from build123d import *

# Parameters (mm, degrees)
SKETCH_1_R      = 1.05
EXTRUDE_1_DEPTH = 1.5
FILLET_1_R      = 1


with BuildPart() as part:
    # 草图1 → 凸台-拉伸1 (new body)
    with BuildSketch(Plane.XY):
        Polygon((23.32, 41.958612035), (27.19, 41.958612035), (27.19, 46.958612035), (24.99, 46.958612035), (24.99, 48.458612035), (29.39, 48.458612035), (29.39, 46.958612035), (28.69, 46.958612035), (28.69, 41.958612035), (33.69, 41.958612035), (33.69, 56.958612035), (14.32, 56.958612035), (-5.05, 56.958612035), (-5.05, 41.958612035), (-0.05, 41.958612035), (-0.05, 46.958612035), (-0.75, 46.958612035), (-0.75, 48.458612035), (3.65, 48.458612035), (3.65, 46.958612035), (1.45, 46.958612035), (1.45, 41.958612035), (5.32, 41.958612035), (5.32, 50.958612035), (23.32, 50.958612035), align=None)
        with Locations((27.94, 53.458612035)):
            Circle(SKETCH_1_R, mode=Mode.SUBTRACT)
        with Locations(Location((0.7, 53.458612035, 0), (0, 0, 180))):
            Circle(SKETCH_1_R, mode=Mode.SUBTRACT)
    extrude(amount=EXTRUDE_1_DEPTH)

    # 圆角1
    fillet_1_edges = [part.edges().sort_by_distance(p)[0] for p in [
        (-5.05, 41.958612035, 0.75),
        (-5.05, 56.958612035, 0.75),
        (33.69, 56.958612035, 0.75),
        (33.69, 41.958612035, 0.75),
        (23.32, 41.958612035, 0.75),
        (5.32, 41.958612035, 0.75),
    ]]
    fillet(fillet_1_edges, radius=FILLET_1_R)


solid = part.part
Input: part model. Units: mm. Frame: model coordinates. A direction names the side the tool comes from. Coordinates: 2 decimals unless noted, no trailing zeros. Loops run counter-clockwise (first coordinate to the right, second up) from the corner with the lowest first, then second, coordinate; pieces in that order, holes last. Notation, with made-up numbers: (12.25, 27.5) -> (64.25, 27.5) arc R23 ccw to (64.25, 43.5) -> close; hole circle Ø9 at (26.25, 14.5). An arc over 180 degrees is marked (long way). One line per item, written item: value.
(1) Set-up query: faces 5 (the face through (24.99, 48, 1)), 6 (the face through (5.32, 47, 1)), 7 (the face through (-4.75, 56.67, 0.76)). Return all of +Z, -Z, +X, -X, +Y, -Y with unobstructed straight access to the full face (end or side cutting, diameter ignored); none if empty.
Answer below:
face 5: +Z, -Z
face 6: +Z, -Z, -Y
face 7: +Z, -Z, -X, +Y
(2) Draft query along X for faces 1 (the face through (-0.05, 44, 1)), 2 (the face through (33.69, 49, 1)), 3 (the face through (-5.05, 50, 1)), 4 (the face through (31, 41.959, 1)). Return one class per face: pulls with the +X half, pulls with the -X half, needs draft (parallel to the pull), parting line crosses it, or undercut.
Answer below:
face 1: undercut
face 2: pulls with the +X half
face 3: pulls with the -X half
face 4: needs draft
(3) Cut plane A-A (y = 46.25). Output: boundary loops of the cut face in (x, z).
Answer below:
outline: (-5.05, 0) -> (-0.05, 0) -> (-0.05, 1.5) -> (-5.05, 1.5) -> close; (1.45, 0) -> (5.32, 0) -> (5.32, 1.5) -> (1.45, 1.5) -> close; (23.32, 0) -> (27.19, 0) -> (27.19, 1.5) -> (23.32, 1.5) -> close; (28.69, 0) -> (33.69, 0) -> (33.69, 1.5) -> (28.69, 1.5) -> close
(4) Pin query (flat end, axial travel): pin 1 Ø1.3 at (x, y) = (27.94, 53.46) entering from -Z. Return the tip coordinate at first contact, or that it passes through.
Answer below:
pin 1: passes through
(5) Ray query, line 1 along X through (y, z) = (47.75, 1.4); line 2 along X through (y, z) = (50.5, 0.45); line 3 along Y through (x, z) = (0.7, 0.9). Return the intervals inside material, ascending.
Answer below:
line 1: x = -5.05 to -0.75, 3.65 to 5.32, 23.32 to 24.99, 29.39 to 33.69
line 2: x = -5.05 to 5.32, 23.32 to 33.69
line 3: y = 48.46 to 52.41, 54.51 to 56.96
(6) Cut plane C-C (x = 0.7). Output: boundary loops of the cut face in (y, z).
Answer below:
outline: (48.46, 0) -> (52.41, 0) -> (52.41, 1.5) -> (48.46, 1.5) -> close; (54.51, 0) -> (56.96, 0) -> (56.96, 1.5) -> (54.51, 1.5) -> close
(7) Cut plane D-D (z = 1.1). Give the number of separate pieces and of enclosed holes in the cut face, then the cut area to 3 significant figures.
Answer below:
separate pieces: 1
enclosed holes: 2
area: 383 mm2
(8) Cut plane B-B (y = 49). Output: boundary loops of the cut face in (x, z).
Answer below:
outline: (-5.05, 0) -> (5.32, 0) -> (5.32, 1.5) -> (-5.05, 1.5) -> close; (23.32, 0) -> (33.69, 0) -> (33.69, 1.5) -> (23.32, 1.5) -> close
